For this review, take the finished solid that the model builds, in its own axes (mm). Face numbers are marked on the shaded views. Give positions to 0.01 mm unless a question says otherwise; leave off trailing zeros. Order: outer loops, then holes, each group sorted by start corner. A loop starts at its lowest first (then second) coordinate and runs counter-clockwise, first axis right, second up.
Item 1: Consider section D-D (x = -5.25). Give the number of separate pieces and of enclosed holes in the cut face, plus the area to 3 significant figures.
Item 2: Consider section B-B (z = 0.3). Give the boundary of the cut face in (x, y).
Item 3: Consider section C-C (y = 6.35). Give the boundary of the cut face in (x, z), plus the area to 3 significant figures.
Item 4: For probe 1 along Y at (x, z) = (0, 1.2); probe 2 along X at (y, z) = (-5.5, 1.8); probe 3 along Y at (x, z) = (0, 2.85), list the stretches that pass through material, from the lowest coordinate up.
Item 5: Consider section A-A (x = 0.5). Give the boundary of the cut face in (y, z), plus the area to 3 significant figures.
Item 6: For P1, Ø1, axis at y = 4, z = 0.5, coming from the -X side, flat-tipped, find the tip position at first contact; note if it passes through.
Item 7: The part is to be moulded in two halves that separate along Y. For the marked faces 1, 2 and 3, say which applies: released by +Y, released by -Y, zero draft, split by the parting line, or undercut.
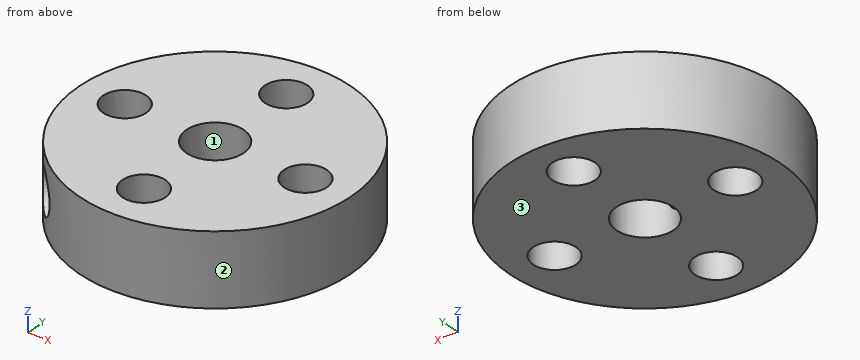
```python
from build123d import *

# Parameters (mm, degrees)
PAD001_DEPTH       = 10
SKETCH007_R        = 1.5
PAD002_DEPTH       = 15
SKETCH_R           = 9.5
PAD_DEPTH          = 5
SKETCH001_R        = 2
POCKET_DEPTH       = 5
SKETCH002_R        = 1.5
POCKET001_DEPTH    = 5
POLARPATTERN_COUNT = 4


with BuildPart() as body001:
    # Sketch006 → Pad001 (new body)
    with BuildSketch(Plane.XY):
        Polygon((-21.213203, 0), (0, -21.213203), (-21.213203, -21.213203), align=None)
    extrude(amount=PAD001_DEPTH)

    # Sketch007 (on Face1 of Pad001) → Pad002 (join)
    with BuildSketch(Plane(origin=(-10.606602, -10.606602, 0), x_dir=(-0.707107, 0.707107, 0), z_dir=(0.707107, 0.707107, 0))):
        with Locations((0, 2.5)):
            Circle(SKETCH007_R)
    extrude(amount=PAD002_DEPTH)


with BuildPart() as body:
    # Sketch → Pad (new body)
    with BuildSketch(Plane.XY):
        Circle(SKETCH_R)
    extrude(amount=PAD_DEPTH)

    # Sketch001 (on Face3 of Pad) → Pocket (cut)
    with BuildSketch(Plane.XY.offset(5)):
        Circle(SKETCH001_R)
    extrude(amount=-POCKET_DEPTH, mode=Mode.SUBTRACT)

    # Sketch002 (on Face3 of Pocket) → Pocket001 (cut)
    with BuildSketch(Plane.XY.offset(5)):
        with Locations((0, 6.35)):
            Circle(SKETCH002_R)
    pocket001 = extrude(amount=-POCKET001_DEPTH, mode=Mode.SUBTRACT)

    # PolarPattern: Pocket001 ×4 about axis
    polarpattern_axis = Axis((0, 0, 5), (0, 0, 1))
    for i in range(1, POLARPATTERN_COUNT):
        add(pocket001.rotate(polarpattern_axis, i * 360 / POLARPATTERN_COUNT), mode=Mode.SUBTRACT)

    # Boolean: cut Body001
    add(body001.part, mode=Mode.SUBTRACT)


solid = body.part
```
Resolved:
1. separate pieces: 2
1. enclosed holes: 1
1. area: 59.0 mm2
2. outline: circle Ø19 at (0, 0); hole circle Ø3 at (-6.35, 0); hole circle Ø4 at (0, 0); hole circle Ø3 at (0, -6.35); hole circle Ø3 at (0, 6.35); hole circle Ø3 at (6.35, 0)
3. outline: (-7.07, 0) - (-1.5, 0) - (-1.5, 5) - (-7.07, 5) - close; (1.5, 0) - (7.07, 0) - (7.07, 5) - (1.5, 5) - close
3. area: 55.7 mm2
4. probe 1: y = -9.5 to -7.85, -4.85 to -2, 2 to 4.85, 7.85 to 9.5
4. probe 2: x = -7.75 to -7.38, -3.62 to -1.24, 1.24 to 7.75
4. probe 3: y = -9.5 to -7.85, -4.85 to -2.06, 2 to 4.85, 7.85 to 9.5
5. outline: (-9.49, 0) - (-7.76, 0) - (-7.76, 5) - (-9.49, 5) - close; (-4.94, 0) - (-1.94, 0) - (-1.94, 5) - (-4.94, 5) - close; (1.94, 0) - (4.94, 0) - (4.94, 5) - (1.94, 5) - close; (7.76, 0) - (9.49, 0) - (9.49, 5) - (7.76, 5) - close
5. area: 47.2 mm2
6. P1: stops at x = -8.83
7. face 1: undercut
7. face 2: split by the parting line
7. face 3: zero draft
